```python
from build123d import *

# Parameters (mm, degrees)
F0_R      = 63.5
F1_DEPTH  = 254
F1_TAPER  = -20
F1_FACE_R = 63.5
F2_DEPTH  = 254
F2_TAPER  = -20
F3_R      = 38.1
F5_T      = -12.7


# Not quite as in the source:
# - a fillet or chamfer that OpenCascade refuses, or shapes differently, is made with other operations: its cross-section is extruded or revolved along the edge and cut away or added
# - a shell that OpenCascade refuses in one call is made with other operations: the cavity is built on its own and cut out


with BuildPart() as f1:
    # F0 (on Front) → F1 (new body)
    with BuildSketch(Plane.XZ):
        Circle(F0_R)
    extrude(amount=F1_DEPTH, taper=F1_TAPER)

    # F1_face (on face) → F2 (join)
    with BuildSketch(Plane(origin=(0, 0, 0), x_dir=(1, 0, 0), z_dir=(0, 1, 0))):
        Circle(F1_FACE_R)
    extrude(amount=F2_DEPTH, taper=F2_TAPER)

    # F3
    f3_edges = [f1.edges().sort_by_distance(p)[0] for p in [
        (-155.94844, -254, 0),
    ]]
    fillet(f3_edges, radius=F3_R)

    # F4: chamfer of 63.5 on 1 edges, made by hand

    # F4_s1 → F4_t2 (revolve, cut)
    with BuildSketch(Plane.XY):
        Polygon((134.2301604024, 194.3295185801), (92.4484395036, 254), (155.9484395036, 254), align=None)
    revolve(axis=Axis((0, 254, 0), (0, -1, 0)), mode=Mode.SUBTRACT)

    # F5: a shell. OpenCascade refuses it in one call, so the cavity is built on its own and cut out:
    # the body offset inwards by the wall thickness, plus a prism from it out through each open face.
    f5_core = offset(f1.part, amount=F5_T, kind=Kind.INTERSECTION, mode=Mode.PRIVATE)
    f5_exits = [f5_core.faces().sort_by_distance(p)[0] for p in [
        (0, -241.3, 0),
    ]]
    add(f5_core, mode=Mode.SUBTRACT)
    extrude(f5_exits, amount=-F5_T, mode=Mode.SUBTRACT)


solid = f1.part
```
Model file for the job. Use its own axes, mm. A direction names the side the tool comes from. Round coordinates to 2 decimals unless told otherwise and drop trailing zeros. Write each loop counter-clockwise with the first axis right and the second up, starting at its lowest first coordinate (ties: lowest second). Pieces come first, ordered by that corner, then holes. Notation, with made-up numbers: (-26, 49) -> (18, 49) arc R10 ccw to (18, 66) -> close; hole circle Ø10 at (61, 62). An arc over 180 degrees is marked (long way). Answer as CSV lines item,"result".
1. Slice it at C-C, the plane x = 0. List the corners of the cut face in (y, z).
Resolved:
outline,"(-254, -101.54) arc R38.1 ccw to (-202.87, -137.34) -> (0, -63.5) -> (194.33, -134.23) -> (254, -92.45) -> (254, 92.45) -> (194.33, 134.23) -> (0, 63.5) -> (-202.87, 137.34) arc R38.1 ccw to (-254, 101.54) -> (-241.3, 101.54) arc R25.4 cw to (-207.21, 125.4) -> (0, 49.98) -> (192.46, 120.03) -> (241.3, 85.84) -> (241.3, -85.84) -> (192.46, -120.03) -> (0, -49.98) -> (-207.21, -125.4) arc R25.4 cw to (-241.3, -101.54) -> close"
2. Drill centre lines: line 1 (Y direction, x = 69, z = 100); line 2 (X direction, y = 97.5, z = 53); line 3 (X direction, y = 205.5, z = -40). Where is each one in solid material? Low to high.
Resolved:
line 1,"-248.35 to -231.61, -196.47 to -159.34, 159.34 to 212.52"
line 2,"-83.6 to -67.06, 67.06 to 83.6"
line 3,"-119.91 to -103.44, 103.44 to 119.91"
3. Mould opens along Y. For faces 1 (the face through (96.847, -247.561, -30.499)), 2 (the face through (-1, 254, -1)), 3 (the face through (-20.102, -80.314, -90.527)) say: +Y half, -Y half, draft (parallel to the pull), parting line (faces both ways), or undercut.
Resolved:
face 1,"draft"
face 2,"+Y half"
face 3,"undercut"
4. Tool access for faces 4 (the face through (-20.481, 251.103, -92.231)), 5 (the face through (-77.64, 76.19, -3.42)): list every direction of +Z, -Z, +X, -X, +Y, -Y with a clear straight run to the whole face (end or side of a thin tool).
Resolved:
face 4,"+Y"
face 5,"none"
5. Slice it at A-A, the plane x = 108. State how many separate pieces and enclosed holes the cut face has, plus the area to 3 significant figures.
Resolved:
separate pieces,"2"
enclosed holes,"2"
area,"16,800 mm²"
6. Pin check, flat tips, straight feed: pin 1 Ø5 at (x, y) = (86.5, -125.5) entering from +Z; pin 2 Ø5 at (x, z) = (-102.5, -84.5) entering from -Y; pin 3 Ø12 at (y, z) = (-130, -62.5) entering from -X. Stop position of each tip, or through.
Resolved:
pin 1,"z = 70.06"
pin 2,"y = -240.84"
pin 3,"x = -96.14"
7. Slice it at D-D, the plane y = -73. List the corners of the cut face in (x, z).
Resolved:
outline,"circle Ø180.14 at (0, 0); hole circle Ø153.11 at (0, 0)"
